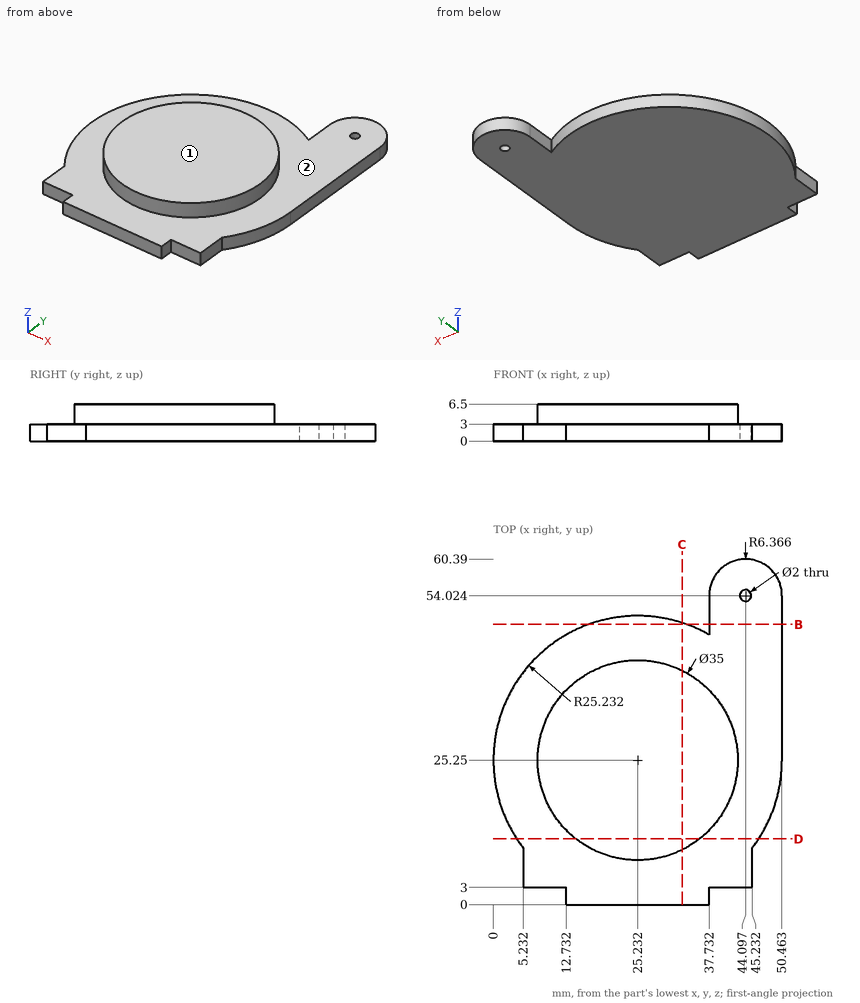
Check sheet for the drawn part. Datum: minimum x, y, z corner. Units: mm. A direction names the side the tool comes from. Round coordinates to 2 decimals unless told otherwise and drop trailing zeros. Order: outer loops, then holes, each group sorted by start corner. A loop starts at its lowest first (then second) coordinate and runs counter-clockwise, first axis right, second up. Notation, with made-up numbers: M -18.5,69.5 L 27.5,69.5 A22 cw 27.5,102.5 Z; hole C 8.5,81.25 d10. An arc over 180 degrees is marked long. Write each question's results on one line, items separated by ' | '. Start each with the question number.
1. Cross-section at C-C on x = 33. Record the boundary of the cut face in (y, z) (1 decimal).
2. Material ranges on L1, parallel to Z at x = 37, y = 45; L2, parallel to X at y = 20.5, z = 1.25; L3, parallel to X at y = 20, z = 1.5, recorded low to high. Write a range as from..to.
3. Go/stop test with flat-tipped pins: P1, Ø3, axis at x = 33, z = 4, coming from the +Y side; P2, Ø1.5, axis at y = 5.5, z = 2, coming from the +X side; P3, Ø3.5, axis at y = 5.5, z = 1, coming from the -X side; P4, Ø1.2, axis at x = 44.1, y = 54.02, coming from the -Z side (3 decimals). Record where each tip stops, or that it passes through.
4. Cross-section at B-B on y = 49. Record the boundary of the cut face in (x, z).
5. Cross-section at D-D on y = 11.5. Record the boundary of the cut face in (x, z) (1 decimal), plus the area to 3 significant figures.
6. Set-up check for the marked faces 1 and 2: record each of +Z, -Z, +X, -X, +Y, -Y from which the full face is reachable in a straight line by a thin tool's end or side.
Resolved:
1) outline: M 0,0 L 49.3,0 L 49.3,3 L 40.9,3 L 40.9,6.5 L 9.6,6.5 L 9.6,3 L 0,3 Z
2) L1: 0..3 | L2: 0.45..50.01 | L3: 0.55..49.91
3) P1: y = 49.59 | P2: x = 45.23 | P3: x = 5.23 | P4: through
4) outline: M 16.71,0 L 33.75,0 L 33.75,3 L 16.71,3 Z; M 37.73,0 L 50.46,0 L 50.46,3 L 37.73,3 Z
5) outline: M 4.1,0 L 46.4,0 L 46.4,3 L 36.1,3 L 36.1,6.5 L 14.4,6.5 L 14.4,3 L 4.1,3 Z | area: 203 mm2
6) face 1: +Z, +X, -X, +Y, -Y | face 2: +Z
